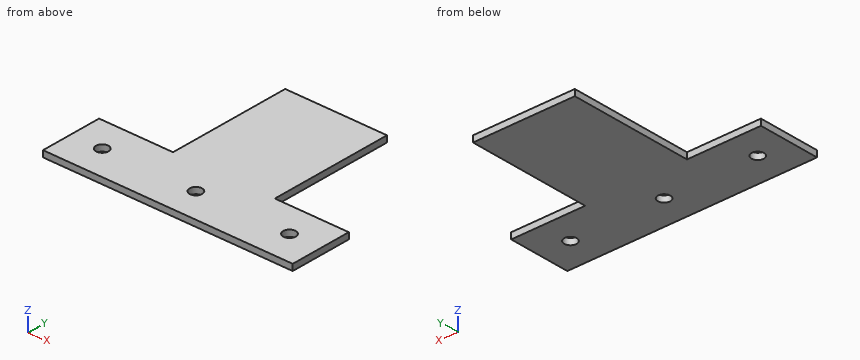
Autodesk Inventor part; units mm, degrees
ref_plane "YZ Plane" through (0, 0, 0) normal (1, 0, 0) x (0, 1, 0)
ref_plane "XZ Plane" through (0, 0, 0) normal (0, 1, 0) x (-1, 0, 0)
ref_plane "XY Plane" through (0, 0, 0) normal (0, 0, 1) x (1, 0, 0)
sketch "Skizze1" plane through (0, 0, 0) normal (0, 0, 1) x (1, 0, 0)
  line L0 (163.1081, -200) -> (163.1081, 0)
  line L1 (163.1081, 0) -> (0, 0)
  line L2 (0, 0) -> (0, -200)
  line L3 (0, -200) -> (-118.4459, -200)
  line L4 (-118.4459, -200) -> (-118.4459, -300)
  line L5 (-118.4459, -300) -> (281.5541, -300)
  line L6 (281.5541, -300) -> (281.5541, -200)
  line L7 (281.5541, -200) -> (163.1081, -200)
  circle A0 centre (231.5541, -250) radius 10
  circle A1 centre (-68.4459, -250) radius 10
  circle A2 centre (81.5541, -250) radius 10
  dimension "d0" = 20
  dimension "d1" = 90
  dimension "d2" = 118.4459
  dimension "d3" = 281.5541
  dimension "d4" = 400
  dimension "d5" = 200
  dimension "d6" = 100
  dimension "d7" = 281.5541
  dimension "d8" = 200
  dimension "d9" = 200
  dimension "d10" = 0
  dimension "d11" = 0
  dimension "d12" = 100
  dimension "d13" = 0
  dimension "d14" = 50
  dimension "d15" = 50
  dimension "d16" = 200
  dimension "d17" = 118.4459
  dimension "d18" = 0
  dimension "d19" = 118.4459
  dimension "d20" = 200
  dimension "d21" = 50
  dimension "d22" = 200
  dimension "d23" = 281.5541
  dimension "d24" = 0
  dimension "d25" = 281.5541
  dimension "d26" = 350
  dimension "d27" = 50
  dimension "d28" = 0
  dimension "d29" = 400
  dimension "d30" = 100
  dimension "d31" = 400
extrude "Extrusion1" add sketch "Skizze1" along normal blind 10
properties part number "aussenOben"
Check sheet for the modelled part. Datum: model origin and axes. Units: mm. Give positions to 0.01 mm unless a question says otherwise; leave off trailing zeros. Write each loop counter-clockwise with the first axis right and the second up, starting at its lowest first coordinate (ties: lowest second). Pieces come first, ordered by that corner, then holes. Notation, with made-up numbers: (57, 39) - (94, 39) arc R25 ccw to (94, 73) - close; hole circle Ø9 at (13, 48). An arc over 180 degrees is marked (long way). Answer as a JSON object with one key per item and string values. Group by question number.
1) Sectioned sample at A-A (y = -250). Record the cut outline in (x, z), then the cut area to 3 significant figures.
2) Sectioned sample at B-B (z = 8). Record the cut outline in (x, y).
3) Thickness scan on probe 1 along X at (y, z) = (-251, 2.5); probe 2 along Y at (x, z) = (82, 3.5); probe 3 along X at (y, z) = (-101, 1.75). Record the ranges inside material, lowest first. Write a range as from..to.
4) Sectioned sample at C-C (x = -71). Record the cut outline in (y, z), then the cut area to 3 significant figures.
5) Sectioned sample at D-D (y = -121). Record the cut outline in (x, z).
6) Depth check by flat-ended pin: P1, Ø3, axis at x = -69.5, z = 3, coming from the +Y side; P2, Ø5, axis at y = -68, z = 5.5, coming from the -X side; P3, Ø18, axis at x = 81.55, y = -250, coming from the +Z side; P4, Ø5, axis at y = -105, z = 6, coming from the +X side. Enter the tip coordinate at first touch or a pass-through.
Geometry results:
{
 "1": {"outline": "(-118.45, 0) - (-78.45, 0) - (-78.45, 10) - (-118.45, 10) - close; (-58.45, 0) - (71.55, 0) - (71.55, 10) - (-58.45, 10) - close; (91.55, 0) - (221.55, 0) - (221.55, 10) - (91.55, 10) - close; (241.55, 0) - (281.55, 0) - (281.55, 10) - (241.55, 10) - close", "area": "3,400 mm^2"},
 "2": {"outline": "(-118.45, -300) - (281.55, -300) - (281.55, -200) - (163.11, -200) - (163.11, 0) - (0, 0) - (0, -200) - (-118.45, -200) - close; hole circle Ø20 at (-68.45, -250); hole circle Ø20 at (81.55, -250); hole circle Ø20 at (231.55, -250)"},
 "3": {"probe 1": "x = -118.45..-78.4, -58.5..71.6, 91.5..221.6, 241.5..281.55", "probe 2": "y = -300..-259.99, -240.01..0", "probe 3": "x = 0..163.11"},
 "4": {"outline": "(-300, 0) - (-259.67, 0) - (-259.67, 10) - (-300, 10) - close; (-240.33, 0) - (-200, 0) - (-200, 10) - (-240.33, 10) - close", "area": "807 mm^2"},
 "5": {"outline": "(0, 0) - (163.11, 0) - (163.11, 10) - (0, 10) - close"},
 "6": {"P1": "stops at y = -200", "P2": "stops at x = 0", "P3": "passes through", "P4": "stops at x = 163.11"}
}
